CAD build for the part. Positions are in the model's coordinates, mm. Face numbers are marked on the shaded views. A direction names the side the tool comes from. Give positions to 0.01 mm unless a question says otherwise; leave off trailing zeros. Answer as a JSON object with one key per item and string values.
```python
from build123d import *

# Parameters (mm, degrees)
SKETCH1_W               = 30
SKETCH1_H               = 15
BOSS_EXTRUDE1_DEPTH     = 5.5
CUT_EXTRUDE2_DEPTH      = 18.649362595
CUT_EXTRUDE2_DEPTH_BACK = 18.649362595
SKETCH2_W               = 0.5
SKETCH2_H               = 0.2
SKETCH7_R               = 6.5
CUT_EXTRUDE6_DEPTH      = 1.75
FILLET1_R               = 1


with BuildPart() as part:
    # Sketch1 → Boss-Extrude1 (new body)
    with BuildSketch(Plane(origin=(0, 0, 0), x_dir=(1, 0, 0), z_dir=(0, 1, 0))):
        Rectangle(SKETCH1_W, SKETCH1_H)
    extrude(amount=BOSS_EXTRUDE1_DEPTH)

    # Sketch2 → Cut-Extrude2 (cut, two sides: drawn at the far end of the back side and taken through both)
    with BuildSketch(Plane(origin=(0, 0, 0), x_dir=(0, 0, -1), z_dir=(1, 0, 0)).offset(-CUT_EXTRUDE2_DEPTH_BACK)):
        with Locations((-5.75, 5.4)):
            Rectangle(SKETCH2_W, SKETCH2_H)
        with Locations((-3.75, 5.4)):
            Rectangle(SKETCH2_W, SKETCH2_H)
        with Locations((-1.75, 5.4)):
            Rectangle(SKETCH2_W, SKETCH2_H)
        with Locations((0.25, 5.4)):
            Rectangle(SKETCH2_W, SKETCH2_H)
        with Locations((2.25, 5.4)):
            Rectangle(SKETCH2_W, SKETCH2_H)
        with Locations((4.25, 5.4)):
            Rectangle(SKETCH2_W, SKETCH2_H)
        with Locations((6.25, 5.4)):
            Rectangle(SKETCH2_W, SKETCH2_H)
    extrude(amount=CUT_EXTRUDE2_DEPTH + CUT_EXTRUDE2_DEPTH_BACK, mode=Mode.SUBTRACT)

    # Sketch8 → Cut-Revolve1 (revolve, cut)
    with BuildSketch(Plane.XY.offset(4), mode=Mode.PRIVATE) as cut_revolve1_sk:
        Polygon((10.25, 0), (10.25, 3), (9, 3.721687836), (9, 0), align=None)
    cut_revolve1 = revolve(cut_revolve1_sk.sketch.rotate(Axis((9, 0, 4), (0, 1, 0)), 90), axis=Axis((9, 0, 4), (0, 1, 0)), mode=Mode.SUBTRACT)

    # Mirror1: Cut-Revolve1 across plane
    add(cut_revolve1.mirror(Plane.XY), mode=Mode.SUBTRACT)

    # Mirror2: Cut-Revolve1 across plane
    add(cut_revolve1.mirror(Plane(origin=(0, 0, 0), x_dir=(0, 0, 1), z_dir=(1, 0, 0))), mode=Mode.SUBTRACT)

    # Mirror2 copy 1 sketch → Mirror2 copy 1 (revolve, cut)
    with BuildSketch(Plane(origin=(0, 0, -4), x_dir=(-1, 0, 0), z_dir=(0, 0, -1))):
        Polygon((10.25, 0), (10.25, 3), (9, 3.721687836), (9, 0), align=None)
    revolve(axis=Axis((-9, 0, -4), (0, 1, 0)), mode=Mode.SUBTRACT)

    # Sketch9 → Cut-Revolve2 (revolve, cut)
    with BuildSketch(Plane.XY, mode=Mode.PRIVATE) as cut_revolve2_sk:
        Polygon((-15, 2.5), (-7.678312164, 2.5), (-8.4, 3.75), (-15, 3.75), align=None)
    revolve(cut_revolve2_sk.sketch.rotate(Axis((-15, 2.5, 0), (-1, 0, 0)), 180), axis=Axis((-15, 2.5, 0), (-1, 0, 0)), mode=Mode.SUBTRACT)

    # Sketch7 → Cut-Extrude6 (cut)
    with BuildSketch(Plane.XZ):
        with Locations((17.59, 0)):
            Circle(SKETCH7_R)
    extrude(amount=-CUT_EXTRUDE6_DEPTH, mode=Mode.SUBTRACT)

    # Fillet1
    fillet1_edges = [part.edges().sort_by_distance(p)[0] for p in [
        (-15, 2.75, -7.5),
        (15, 2.75, -7.5),
        (15, 2.75, 7.5),
        (-15, 2.75, 7.5),
    ]]
    fillet(fillet1_edges, radius=FILLET1_R - 0.0001)  # a hair under: the kernel refuses the full size


solid = part.part
```
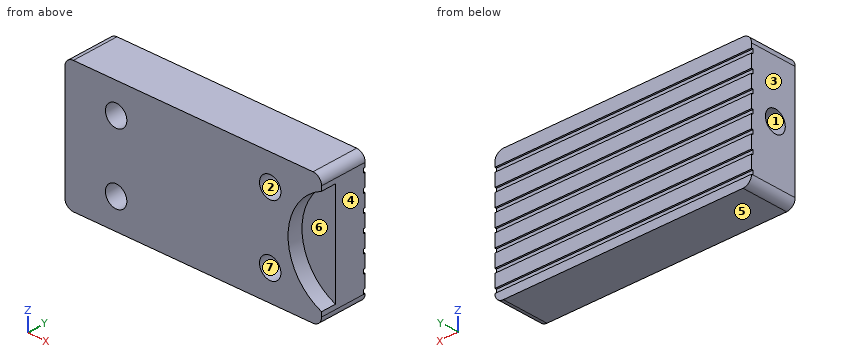
1) 3-axis set-ups, long thin cutter, end or side, ignore diameter. For the marked faces 1, 2 and 3: which of +Z, -Z, +X, -X, +Y, -Y reach the whole face in a straight line?
Model answer:
{"face 1": "-X", "face 2": "-Y", "face 3": "+Z, -Z, -X, +Y, -Y"}
2) Pin check, flat tips, straight feed: pin 1 (1.5 mm diameter, centred on y = 2.5, z = 0, fed in from -X); pin 2 (2 mm diameter, centred on x = -9, z = -4, fed in from -Y). Stop position of each tip, or through.
Model answer:
{"pin 1": "stops at x = -8.11", "pin 2": "stops at y = 3.14"}
3) Mould opens along Z. For the marked faces 4, 5, 6 and 7 say: released by +Z, released by -Z, zero draft, split by the parting line, or undercut.
Model answer:
{"face 4": "zero draft", "face 5": "released by -Z", "face 6": "undercut", "face 7": "undercut"}
4) Wall check: probe 1 along X at (y, z) = (1.3, 4); probe 2 along Z at (x, y) = (-12.5, 2.5); probe 3 along X at (y, z) = (0.8, -4.75). Give the ranges that are in metal, low to high.
Model answer:
{"probe 1": "x = -15 to -10.25, -7.75 to 7.75, 10.25 to 12.47", "probe 2": "z = -7.5 to -1.25, 1.25 to 7.5", "probe 3": "x = -15 to -10, -8 to 8, 10 to 13.15"}
